from build123d import *

# Parameters (mm, degrees)
BOSS_EXTRUDE1_DEPTH = 8.7
BOSS_EXTRUDE3_START = 8.7
SKETCH1_3_R         = 0.5
BOSS_EXTRUDE3_DEPTH = 38.2
SKETCH2_3_W         = 0.5
SKETCH2_3_H         = 10.1
BOSS_EXTRUDE4_DEPTH = 6.05
FILLET2_SIZE        = 5
FILLET2_SIZE_2      = 2
SKETCH2_W           = 1
SKETCH2_H           = 10
SKETCH2_H_2         = 7
BOSS_EXTRUDE2_DEPTH = 6
FILLET1_R           = 1
SKETCH2_5_W         = 2
SKETCH2_5_H         = 5.05
SKETCH3_R           = 2
BOSS_EXTRUDE5_DEPTH = 0.5
SKETCH4_W           = 8
SKETCH4_H           = 2.95
SKETCH4_H_2         = 1.05
BOSS_EXTRUDE6_DEPTH = 0.55


with BuildPart() as part:
    # Sketch1 → Boss-Extrude1 (new body)
    with BuildSketch(Plane.XY):
        with BuildLine():
            Line((1, 1.118033989), (-1, 1.118033989))
            ThreePointArc((-1, 1.118033989), (0, -1.5), (1, 1.118033989))
        make_face()
    extrude(amount=BOSS_EXTRUDE1_DEPTH)

    # Sketch1<3> → Boss-Extrude3 (add)
    with BuildSketch(Plane.XY.offset(BOSS_EXTRUDE3_START)):
        Circle(SKETCH1_3_R)
    extrude(amount=-BOSS_EXTRUDE3_DEPTH)

    # Sketch2<3> → Boss-Extrude4 (add, symmetric)
    with BuildSketch(Plane(origin=(0, 0, 0), x_dir=(0, 0, -1), z_dir=(1, 0, 0))):
        Polygon((9.5, 5.05), (9.5, 5), (9.5, -5), (9.5, -5.05), (24.5, -5.05), (24.5, 0), (24.5, 5.05), align=None)
        with Locations((26, 0)):
            Rectangle(SKETCH2_3_W, SKETCH2_3_H)
    extrude(amount=BOSS_EXTRUDE4_DEPTH, both=True)

    # Fillet2
    # an asymmetric fillet: 5, 2 mm, written as the material it takes off along each edge
    with BuildSketch(Plane(origin=(-6.05, -5.05, 3), x_dir=(0, 1, 0), z_dir=(0, 0, -1)), Plane(origin=(-6.05, 5.05, -37), x_dir=(0, -1, 0), z_dir=(0, 0, 1))) as fillet2_piece_1:
        with BuildLine():
            Bezier((FILLET2_SIZE, 0), (0, 0), (0, FILLET2_SIZE_2), weights=[1, 0.707106781, 1])
            Line((0, FILLET2_SIZE_2), (0, 0))
            Line((0, 0), (FILLET2_SIZE, 0))
        make_face()
    extrude(amount=40, mode=Mode.SUBTRACT)
    with BuildSketch(Plane(origin=(6.05, -5.05, 3), x_dir=(-1, 0, 0), z_dir=(0, 0, -1)), Plane(origin=(6.05, 5.05, -37), x_dir=(-1, 0, 0), z_dir=(0, 0, 1))) as fillet2_piece_2:
        with BuildLine():
            Bezier((FILLET2_SIZE_2, 0), (0, 0), (0, FILLET2_SIZE), weights=[1, 0.707106781, 1])
            Line((0, FILLET2_SIZE), (0, 0))
            Line((0, 0), (FILLET2_SIZE_2, 0))
        make_face()
    extrude(amount=40, mode=Mode.SUBTRACT)
    with BuildSketch(Plane(origin=(-6.05, -5.05, -13.25), x_dir=(0, 1, 0), z_dir=(0, 0, -1)), Plane(origin=(-6.05, 5.05, -38.75), x_dir=(0, -1, 0), z_dir=(0, 0, 1))) as fillet2_piece_3:
        with BuildLine():
            Bezier((FILLET2_SIZE, 0), (0, 0), (0, FILLET2_SIZE_2), weights=[1, 0.707106781, 1])
            Line((0, FILLET2_SIZE_2), (0, 0))
            Line((0, 0), (FILLET2_SIZE, 0))
        make_face()
    extrude(amount=25.5, mode=Mode.SUBTRACT)
    with BuildSketch(Plane(origin=(6.05, -5.05, -13.25), x_dir=(-1, 0, 0), z_dir=(0, 0, -1)), Plane(origin=(6.05, 5.05, -38.75), x_dir=(-1, 0, 0), z_dir=(0, 0, 1))) as fillet2_piece_4:
        with BuildLine():
            Bezier((FILLET2_SIZE_2, 0), (0, 0), (0, FILLET2_SIZE), weights=[1, 0.707106781, 1])
            Line((0, FILLET2_SIZE), (0, 0))
            Line((0, 0), (FILLET2_SIZE_2, 0))
        make_face()
    extrude(amount=25.5, mode=Mode.SUBTRACT)

    # Sketch2 → Boss-Extrude2 (add, symmetric)
    with BuildSketch(Plane(origin=(0, 0, 0), x_dir=(0, 0, -1), z_dir=(1, 0, 0))):
        with Locations((1, 0)):
            Rectangle(SKETCH2_W, SKETCH2_H)
        with Locations((3.666666667, -1.5)):
            Rectangle(SKETCH2_W, SKETCH2_H_2)
        with Locations((9, 0)):
            Rectangle(SKETCH2_W, SKETCH2_H)
        with Locations((6.333333333, 0)):
            Rectangle(SKETCH2_W, SKETCH2_H)
    extrude(amount=BOSS_EXTRUDE2_DEPTH, both=True)

    # Fillet1
    fillet1_edges = [part.edges().sort_by_distance(p)[0] for p in [
        (-6, 5, -1),
        (6, 5, -1),
        (-6, -5, -1),
        (-6, -5, -3.666666667),
        (-6, -5, -6.333333333),
        (-6, -5, -9),
        (-6, 5, -9),
        (-6, 5, -6.333333333),
        (-6, 2, -3.666666667),
        (6, 5, -9),
        (6, 5, -6.333333333),
        (6, 2, -3.666666667),
        (6, -5, -9),
        (6, -5, -6.333333333),
        (6, -5, -3.666666667),
        (6, -5, -1),
    ]]
    fillet(fillet1_edges, radius=FILLET1_R)

    # Sketch2<5> → Revolve1 (revolve)
    with BuildSketch(Plane(origin=(0, 0, 0), x_dir=(0, 0, -1), z_dir=(1, 0, 0))):
        with Locations((28.5, 2.525)):
            Rectangle(SKETCH2_5_W, SKETCH2_5_H)
    revolve(axis=Axis((0, 0, -27.5), (0, 0, -1)))

    # Sketch3 → Boss-Extrude5 (add)
    with BuildSketch(Plane.XY.offset(-0.5)):
        with Locations(Location((0, 0, 0), (0, 0, 180))):
            Circle(SKETCH3_R)
    extrude(amount=BOSS_EXTRUDE5_DEPTH)

    # Sketch4 → Boss-Extrude6 (add, symmetric)
    with BuildSketch(Plane.XY.offset(-25.75)):
        with Locations((0, -6.525)):
            Rectangle(SKETCH4_W, SKETCH4_H)
        with Locations((0, -4.525)):
            Rectangle(SKETCH4_W, SKETCH4_H_2)
    extrude(amount=BOSS_EXTRUDE6_DEPTH, both=True)


solid = part.part
The listing builds one solid part. Answer for the finished solid, in the listing's coordinates (mm). A direction names the side the tool comes from. Give positions to 0.01 mm unless a question says otherwise; leave off trailing zeros. Write each loop counter-clockwise with the first axis right and the second up, starting at its lowest first coordinate (ties: lowest second). Pieces come first, ordered by that corner, then holes. Notation, with made-up numbers: (76, 8) - (100, 8) arc R12 cw to (100, 14) - close; hole circle Ø8 at (-17, -5). An arc over 180 degrees is marked (long way). Use a Markdown table: item, result.
1. Each of these flat-tipped pins is pushed along its axis until it touches: P1, Ø4, axis at y = -2, z = -1, coming from the -X side; P2, Ø1, axis at x = -2.5, z = -3.5, coming from the +Y side; P3, Ø1.5, axis at x = 1, z = 1.5, coming from the -Y side. Where does it stop, or does it pass through?
Values follow:
| item | result |
|---|---|
| P1 | stops at x = -6 |
| P2 | stops at y = 2 |
| P3 | stops at y = -1.48 |
2. For a pull along Z with two mould halves and no side action, classify faces 4 (the cylindrical face through (-0.108, -0.488, -7.655)), 5 (the flat face through (-0.1, 2.2, -0.5)), 6 (the flat face through (0, 1.118, 4)) as released by +Z, released by -Z, zero draft, split by the parting line, or undercut.
Values follow:
| item | result |
|---|---|
| face 4 | undercut |
| face 5 | released by +Z |
| face 6 | zero draft |
3. Section C-C on z = 1 is taken. Write down the section's boundary in (x, y), plus the area to 3 significant figures.
Values follow:
| item | result |
|---|---|
| outline | (-1, 1.12) arc R1.5 ccw (long way) to (1, 1.12) - close |
| area | 6.54 mm² |
4. Find the intervals of material crossed by probe 1 along Z at (x, y) = (-4.5, -3.25); probe 2 along Z at (x, y) = (1.25, 0.5); probe 3 along Z at (x, y) = (2.5, -4.25), in increasing order. Write a range as from..to.
Values follow:
| item | result |
|---|---|
| probe 1 | z = -26.25..-25.75, -24.5..-8.5, -6.83..-5.83, -4.17..-3.17, -1.5..-0.5 |
| probe 2 | z = -29.5..-27.5, -26.25..-25.75, -24.5..-8.5, -6.83..-5.83, -4.17..-3.17, -1.5..8.7 |
| probe 3 | z = -29.5..-27.5, -26.3..-25.2, -24.5..-8.5, -6.83..-5.83, -4.17..-3.17, -1.5..-0.5 |
5. Section A-A on x = 2.5 is taken. Count the separate pieces of the cut face and the enclosed holes in it, plus the area to 3 significant figures.
Values follow:
| item | result |
|---|---|
| separate pieces | 6 |
| enclosed holes | 0 |
| area | 215 mm² |
6. Section B-B on y = -6.5 is taken. Write down the section's boundary in (x, z), plus the area to 3 significant figures.
Values follow:
| item | result |
|---|---|
| outline | (-4, -26.3) - (4, -26.3) - (4, -25.2) - (-4, -25.2) - close |
| area | 8.80 mm² |
7. A tool of negligible diameter and unlimited length cuts with its end or side. For faces 1 (the cylindrical face through (-0.108, -0.488, -25.116)), 2 (the flat face through (0, 5, -9)), 3 (the flat face through (0, -5.05, -17)), from which of +Z, -Z, +X, -X, +Y, -Y can it reach the whole face along a straight path? Write none if from no direction.
Values follow:
| item | result |
|---|---|
| face 1 | none |
| face 2 | +Z, +X, -X, +Y |
| face 3 | +Z, +X, -X, -Y |
